from build123d import *

# Parameters (mm, degrees)
SKETCH1_R             = 14
SKETCH1_R_2           = 10.16
BOSS_EXTRUDE1_DEPTH   = 5
SKETCH1_3_W           = 40
SKETCH1_3_H           = 40
SKETCH1_3_R           = 14
BOSS_EXTRUDE2_DEPTH   = 1
CUT_EXTRUDE1_START    = -4
SKETCH2_R             = 14
SKETCH2_R_2           = 12
CUT_EXTRUDE1_DEPTH    = 4
SKETCH3_W             = 1
SKETCH3_H             = 40
BOSS_EXTRUDE3_DEPTH   = 50
BOSS_EXTRUDE5_DEPTH   = 50
SKETCH5_W             = 40
SKETCH5_H             = 50
CUT_EXTRUDE2_DEPTH    = 22
M2_TAPPED_HOLE2_D     = 1.6
M2_TAPPED_HOLE2_DEPTH = 6
M2_TAPPED_HOLE2_TIP   = 0.480688495


with BuildPart() as part:
    # Sketch1 → Boss-Extrude1 (new body)
    with BuildSketch(Plane(origin=(0, 0, 0), x_dir=(0, 1, 0), z_dir=(0, 0, 1))):
        with Locations(Location((0, 0, 0), (0, 0, 270))):
            Circle(SKETCH1_R)
        with Locations(Location((0, 0, 0), (0, 0, 270))):
            Circle(SKETCH1_R_2, mode=Mode.SUBTRACT)
    extrude(amount=BOSS_EXTRUDE1_DEPTH)

    # Sketch1<3> → Boss-Extrude2 (add)
    with BuildSketch(Plane(origin=(0, 0, 0), x_dir=(0, 1, 0), z_dir=(0, 0, 1))):
        Rectangle(SKETCH1_3_W, SKETCH1_3_H)
        with Locations(Location((0, 0, 0), (0, 0, 270))):
            Circle(SKETCH1_3_R, mode=Mode.SUBTRACT)
    extrude(amount=BOSS_EXTRUDE2_DEPTH)

    # Sketch2 → Cut-Extrude1 (cut)
    with BuildSketch(Plane.XY.offset(5).offset(CUT_EXTRUDE1_START)):
        Circle(SKETCH2_R)
        Circle(SKETCH2_R_2, mode=Mode.SUBTRACT)
    extrude(amount=CUT_EXTRUDE1_DEPTH, mode=Mode.SUBTRACT)

    # Sketch3 → Boss-Extrude3 (add)
    with BuildSketch(Plane.XY.offset(1)):
        with Locations((-19.5, 0)):
            Rectangle(SKETCH3_W, SKETCH3_H)
    extrude(amount=BOSS_EXTRUDE3_DEPTH)

    # Sketch4 → Boss-Extrude5 (add)
    with BuildSketch(Plane.XY.offset(51)):
        Polygon((-17, 5), (-19, 4), (-19, 0), (-19, -4), (-17, -5), align=None)
    extrude(amount=-BOSS_EXTRUDE5_DEPTH)

    # Sketch5 → Cut-Extrude2 (cut)
    with BuildSketch(Plane.YZ.offset(-17)):
        with Locations((0, 26)):
            Rectangle(SKETCH5_W, SKETCH5_H)
    extrude(amount=-CUT_EXTRUDE2_DEPTH, mode=Mode.SUBTRACT)

    # M2 Tapped Hole2
    with Locations(Plane.XY.offset(1)):
        with Locations((-16.5, -16.5), (-16.5, 16.5), (16.5, 16.5), (16.5, -16.5)):
            Hole(M2_TAPPED_HOLE2_D / 2, depth=M2_TAPPED_HOLE2_DEPTH)
            with Locations((0, 0, -(M2_TAPPED_HOLE2_DEPTH + M2_TAPPED_HOLE2_TIP / 2))):  # 118° drill point
                Cone(0, M2_TAPPED_HOLE2_D / 2, M2_TAPPED_HOLE2_TIP, mode=Mode.SUBTRACT)


solid = part.part
Could you check a few things on this model? Use its own coordinates, in mm. A direction names the side the tool comes from. Give positions to 0.01 mm unless a question says otherwise; leave off trailing zeros. Order: outer loops, then holes, each group sorted by start corner. A loop starts at its lowest first (then second) coordinate and runs counter-clockwise, first axis right, second up.
1. I need wall thicknesses on L1, parallel to Y at x = -16.5, z = 0.7; L2, parallel to Y at x = 7.5, z = 0.45; L3, parallel to Y at x = 7, z = 4.35. Which ranges of each line are inside material? Lowest first, please.
2. Suppose I cut it at C-C (y = 16.5). List the corners of the cut face in (x, z) for me.
3. For faces 1 (the cylindrical face through (-1.323, 10.074, 2.465)), 2 (the flat face through (9, 9, 1)), which set-ups out of +Z, -Z, +X, -X, +Y, -Y let a thin tool reach every point of the face, with its end or its side?
4. Will these pins go through, and if not, where does the flat tip stop? P1, Ø1, axis at x = -16.5, y = 16.5, coming from the -Z side; P2, Ø2, axis at x = 12.5, y = -7, coming from the +Z side; P3, Ø1.5, axis at y = 5, z = 3.5, coming from the -X side; P4, Ø1.5, axis at x = 3.5, z = 2, coming from the -Y side.
5. Suppose I cut it at A-A (y = 0). List the corners of the cut face in (x, z) for me, plus the area to 3 significant figures.
6. We'd pull the mould along X, two halves only. Please class faces 3 (the flat face through (-20, -0.3, 0.5)), 4 (the cylindrical face through (-15.87, -16.99, 0.49)), 5 (the flat face through (-0.3, -20, 0.5)), 6 (the cylindrical face through (-11.99, 0.53, 2.97)): pulls with the +X half, pulls with the -X half, needs draft (parallel to the pull), parting line crosses it, or undercut.
Solved:
1. L1: y = -20 to -17.3, -15.7 to 15.7, 17.3 to 20
1. L2: y = -20 to -6.85, 6.85 to 20
1. L3: y = -9.75 to -7.36, 7.36 to 9.75
2. outline: (-20, 0) - (-17.3, 0) - (-17.3, 1) - (-20, 1) - close; (-15.7, 0) - (15.7, 0) - (15.7, 1) - (-15.7, 1) - close; (17.3, 0) - (20, 0) - (20, 1) - (17.3, 1) - close
3. face 1: +Z, -Z
3. face 2: +Z
4. P1: passes through
4. P2: stops at z = 1
4. P3: stops at x = -11.22
4. P4: stops at y = -11.68
5. outline: (-20, 0) - (-10.16, 0) - (-10.16, 5) - (-12, 5) - (-12, 1) - (-20, 1) - close; (10.16, 0) - (20, 0) - (20, 1) - (12, 1) - (12, 5) - (10.16, 5) - close
5. area: 34.4 mm2
6. face 3: pulls with the -X half
6. face 4: undercut
6. face 5: needs draft
6. face 6: parting line crosses it
